from build123d import *

# Parameters (mm, degrees)
BOSS_EXTRUDE1_DEPTH = 6.75
SKETCH3_R           = 8
CUT_EXTRUDE2_DEPTH  = 3
SKETCH4_W           = 27
SKETCH4_H           = 2
CUT_EXTRUDE3_DEPTH  = 9
SKETCH5_R           = 1.5
CUT_EXTRUDE4_DEPTH  = 16
FILLET1_R           = 4


with BuildPart() as part:
    # Sketch1 → Boss-Extrude1 (new body)
    with BuildSketch(Plane.XY):
        with BuildLine():
            Line((-27, 0), (0, 0))
            Line((0, 0), (0, 12.5))
            Line((0, 12.5), (-7.5, 12.5))
            ThreePointArc((-7.5, 12.5), (-13.5, 6.5), (-19.5, 12.5))
            Line((-19.5, 12.5), (-27, 12.5))
            Line((-27, 12.5), (-27, 0))
        make_face()
    extrude(amount=BOSS_EXTRUDE1_DEPTH)

    # Sketch3 → Cut-Extrude2 (cut)
    with BuildSketch(Plane(origin=(0, 0, 0), x_dir=(-1, 0, 0), z_dir=(0, 0, -1))):
        with Locations((13.5, 12.5)):
            Circle(SKETCH3_R)
    extrude(amount=-CUT_EXTRUDE2_DEPTH, mode=Mode.SUBTRACT)

    # Sketch4 → Cut-Extrude3 (cut)
    with BuildSketch(Plane.XY.offset(6.75)):
        with Locations((-13.5, 11.5)):
            Rectangle(SKETCH4_W, SKETCH4_H)
    extrude(amount=-CUT_EXTRUDE3_DEPTH, mode=Mode.SUBTRACT)

    # Sketch5 → Cut-Extrude4 (cut)
    with BuildSketch(Plane.XZ):
        with Locations((-23.5, 3.375)):
            Circle(SKETCH5_R)
        with Locations((-3.5, 3.375)):
            Circle(SKETCH5_R)
    extrude(amount=-CUT_EXTRUDE4_DEPTH, mode=Mode.SUBTRACT)

    # Fillet1
    # the kernel refuses this fillet: 4 mm, written as the material it takes off along each edge
    with BuildSketch(Plane(origin=(-27, 10.5, 16.75), x_dir=(1, 0, 0), z_dir=(0, 0, -1))) as fillet1_piece_1:
        with BuildLine():
            CenterArc((FILLET1_R, FILLET1_R), FILLET1_R, 180, 90)
            Line((0, FILLET1_R), (0, 0))
            Line((0, 0), (FILLET1_R, 0))
        make_face()
    extrude(amount=26.75, mode=Mode.SUBTRACT)
    with BuildSketch(Plane(origin=(0, 10.5, 16.75), x_dir=(-1, 0, 0), z_dir=(0, 0, -1))) as fillet1_piece_2:
        with BuildLine():
            CenterArc((FILLET1_R, -FILLET1_R), FILLET1_R, 90, 90)
            Line((0, -FILLET1_R), (0, 0))
            Line((0, 0), (FILLET1_R, 0))
        make_face()
    extrude(amount=26.75, mode=Mode.SUBTRACT)


solid = part.part
The listing builds one solid part. Answer for the finished solid, in the listing's coordinates (mm). A direction names the side the tool comes from. Coordinates: 2 decimals unless noted, no trailing zeros. Loops run counter-clockwise (first coordinate to the right, second up) from the corner with the lowest first, then second, coordinate; pieces in that order, holes last. Notation, with made-up numbers: (-30.75, -31) -> (27.25, -31) arc R28 cw to (27.25, -10) -> close; hole circle Ø7 at (13, 83). An arc over 180 degrees is marked (long way). Answer in a Markdown table with one row per item. Add a question column.
1. Determine the mould class of faces 1 (the flat face through (-14, 4, 6.75)), 2 (the cylindrical face through (-2.07, 5.18, 3.83)), 3 (the flat face through (-14, 0, 3)), 4 (the cylindrical face through (-25, 5.2, 3.4)) for opening direction Z: +Z half, -Z half, draft (parallel to the pull), parting line (faces both ways), or undercut.
2. The part is cut by section C-C, the plane x = -23.5. Write down the section's boundary in (y, z) (3 decimals), then the cut area to 3 significant figures.
3. Consider line 1 (X direction, y = 1.5, z = 3.25); line 2 (Z direction, x = -3.5, y = 8.5) (3 decimals); line 3 (X direction, y = 9, z = 4.5). Determine where each line is inside the solid, lowest interval first. Write a range as [from, to].
4. The part is cut by section B-B, the plane y = 8.25. Write down the section's boundary in (x, z) (3 decimals), then the cut area to 3 significant figures.
5. For faces 5 (the cylindrical face through (-13.4, 4.5, 1.5)), 6 (the flat face through (-21, 10.5, 4)), determine the directions among +Z, -Z, +X, -X, +Y, -Y from which every point of the face is accessible in a straight line to the end or side of a thin tool.
6. The part is cut by section D-D, the plane z = 0.5. Write down the section's boundary in (x, y).
7. Flat-ended cylindrical pins translate along their axes: P1, Ø3, axis at x = -10.5, y = 8.5, coming from the -Z side; P2, Ø1, axis at x = -3.5, z = 3.5, coming from the -Y side. Find the tip coordinate at first contact, or state that the pin passes through.
8. The part is cut by section A-A, the plane z = 4. Write down the section's boundary in (x, y).
Answer below:
| question | item | result |
|---|---|---|
| 1 | face 1 | +Z half |
| 1 | face 2 | undercut |
| 1 | face 3 | draft |
| 1 | face 4 | undercut |
| 2 | outline | (0, 0) -> (10.469, 0) -> (10.469, 1.875) -> (0, 1.875) -> close; (0, 4.875) -> (10.469, 4.875) -> (10.469, 6.75) -> (0, 6.75) -> close |
| 2 | area | 39.3 mm2 |
| 3 | line 1 | [-27, -24.99], [-22.01, -4.99], [-2.01, 0] |
| 3 | line 2 | [0, 1.875], [4.875, 6.75] |
| 3 | line 3 | [-26.12, -24.49], [-22.51, -18.37], [-8.63, -4.49], [-2.51, -0.88] |
| 4 | outline | (-26.597, 0) -> (-20.278, 0) -> (-20.278, 3) -> (-17.735, 3) -> (-17.735, 6.75) -> (-26.597, 6.75) -> close; (-9.265, 3) -> (-6.722, 3) -> (-6.722, 0) -> (-0.403, 0) -> (-0.403, 6.75) -> (-9.265, 6.75) -> close; hole circle Ø3 at (-23.5, 3.375); hole circle Ø3 at (-3.5, 3.375) |
| 4 | area | 90.2 mm2 |
| 5 | face 5 | -Z, +Y |
| 5 | face 6 | +Z, -Z, +X, -X, +Y |
| 6 | outline | (-27, 0) -> (0, 0) -> (0, 6.5) arc R4 ccw to (-4, 10.5) -> (-5.75, 10.5) arc R8 cw to (-21.25, 10.5) -> (-23, 10.5) arc R4 ccw to (-27, 6.5) -> close |
| 7 | P1 | z = 3 |
| 7 | P2 | through |
| 8 | outline | (-27, 0) -> (-24.86, 0) -> (-24.86, 10.04) arc R4 ccw to (-27, 6.5) -> close; (-22.14, 0) -> (-4.86, 0) -> (-4.86, 10.5) -> (-7.84, 10.5) arc R6 cw to (-19.16, 10.5) -> (-22.14, 10.5) -> close; (-2.14, 0) -> (0, 0) -> (0, 6.5) arc R4 ccw to (-2.14, 10.04) -> close |
